Geometry: final body of the model. Coordinates: model frame, mm. A direction names the side the tool comes from. Give positions to 0.01 mm unless a question says otherwise; leave off trailing zeros. Write each loop counter-clockwise with the first axis right and the second up, starting at its lowest first coordinate (ties: lowest second). Pieces come first, ordered by that corner, then holes. Notation, with made-up numbers: M -7.75,7.5 L -0.75,7.5 A12 cw -0.75,28.5 Z; hole C 22,9 d4. An arc over 180 degrees is marked long. Use a Markdown table: item, result. Add a question column.
1) Section A-A on x = 4.75. Return the cut outline in (y, z).
2) Set-up query: faces 1 (the cylindrical face through (24.012, 12.918, 14.087)), 2 (the flat face through (19.05, -19, -5)), 3 (the cylindrical face through (23.638, -25.238, -13.127)). Return all of +Z, -Z, +X, -X, +Y, -Y with unobstructed straight access to the full face (end or side cutting, diameter ignored); none if empty.
3) Draft query along Y for faces 4 (the conical face through (19.2, -18.96, -9.86)), 5 (the flat face through (23.368, -6, -17)), 6 (the flat face through (0, -6, -17)). Return one class per face: +Y half, -Y half, draft (parallel to the pull), parting line (faces both ways), or undercut.
4) Pin query (flat end, axial travel): pin 1 (3 mm diameter, centred on y = 22.5, z = 3.5, fed in from -X); pin 2 (5 mm diameter, centred on x = 19.5, z = -3.5, fed in from -Y); pin 3 (10 mm diameter, centred on x = 17, y = -8.5, fed in from -Z). Return the tip coordinate at first contact, or that it passes through.
5) Line query: line 1 (Y direction, x = 23.65, z = 0); line 2 (Y direction, x = 10.25, z = 0); line 3 (Z direction, x = 12.25, y = 0.5). Output: solid intervals per line, ascending.
```python
from build123d import *

# Parameters (mm, degrees)
SKETCH1_R           = 19.05
SKETCH1_R_2         = 17.526
BOSS_EXTRUDE1_DEPTH = 19.05
SKETCH2_R           = 28.448
BOSS_EXTRUDE2_DEPTH = 5.588
CHAMFER1_SIZE       = 7.493
CHAMFER1_SIZE2      = 2.727228965
FILLET2_R           = 1.27
SKETCH3_R           = 17.526
CUT_EXTRUDE1_DEPTH  = 6.5880001
SKETCH4_R           = 19.1135
SKETCH4_R_2         = 17.526
CUT_EXTRUDE2_DEPTH  = 1.27


with BuildPart() as part:
    # Sketch1 → Boss-Extrude1 (new body)
    with BuildSketch(Plane(origin=(0, 0, 0), x_dir=(0, 0, -1), z_dir=(1, 0, 0))):
        Circle(SKETCH1_R)
        Circle(SKETCH1_R_2, mode=Mode.SUBTRACT)
    extrude(amount=BOSS_EXTRUDE1_DEPTH)

    # Sketch2 → Boss-Extrude2 (add)
    with BuildSketch(Plane(origin=(19.05, 0, 0), x_dir=(0, 0, -1), z_dir=(1, 0, 0))):
        Circle(SKETCH2_R)
    extrude(amount=BOSS_EXTRUDE2_DEPTH)

    # Chamfer1
    chamfer1_edges = [part.edges().sort_by_distance(p)[0] for p in [
        (19.05, 0, 28.448),
    ]]
    chamfer1_side = [part.faces().sort_by_distance(p)[0] for p in [
        (19.05, 0, 27.643369052),
    ]]
    chamfer(chamfer1_edges, length=CHAMFER1_SIZE, length2=CHAMFER1_SIZE2, reference=chamfer1_side[0])

    # Fillet2
    fillet2_edges = [part.edges().sort_by_distance(p)[0] for p in [
        (21.777228965, 0, 28.448),
    ]]
    fillet(fillet2_edges, radius=FILLET2_R)

    # Sketch3 → Cut-Extrude1 (cut, through all)
    with BuildSketch(Plane.ZY.offset(-19.05)):
        Circle(SKETCH3_R)
    extrude(amount=-CUT_EXTRUDE1_DEPTH, mode=Mode.SUBTRACT)

    # Sketch4 → Cut-Extrude2 (cut)
    with BuildSketch(Plane(origin=(24.638, 0, 0), x_dir=(0, 0, -1), z_dir=(1, 0, 0))):
        Circle(SKETCH4_R)
        Circle(SKETCH4_R_2, mode=Mode.SUBTRACT)
    extrude(amount=-CUT_EXTRUDE2_DEPTH, mode=Mode.SUBTRACT)


solid = part.part
```
Found:
| question | item | result |
|---|---|---|
| 1 | outline | C 0,0 d38.1; hole C 0,0 d35.05 |
| 2 | face 1 | +X |
| 2 | face 2 | -X |
| 2 | face 3 | +X, -X |
| 3 | face 4 | parting line |
| 3 | face 5 | undercut |
| 3 | face 6 | draft |
| 4 | pin 1 | x = 19.16 |
| 4 | pin 2 | y = -28.07 |
| 4 | pin 3 | z = -27.2 |
| 5 | line 1 | -28.45 to -19.11, 19.11 to 28.45 |
| 5 | line 2 | -19.05 to -17.53, 17.53 to 19.05 |
| 5 | line 3 | -19.04 to -17.52, 17.52 to 19.04 |
